Check sheet for the modelled part. Datum: model origin and axes. Units: mm. Face numbers are marked on the shaded views. Round coordinates to 2 decimals unless told otherwise and drop trailing zeros. Write each loop counter-clockwise with the first axis right and the second up, starting at its lowest first coordinate (ties: lowest second). Pieces come first, ordered by that corner, then holes. Notation, with made-up numbers: M 45.25,25.5 L 53.25,25.5 A18 ccw 53.25,49.5 Z; hole C 50.5,-20.75 d7. An arc over 180 degrees is marked long. Put each result on its own line as item: value.
Autodesk Inventor part; units mm, degrees
ref_plane "YZ Plane" through (0, 0, 0) normal (1, 0, 0) x (0, 1, 0)
ref_plane "XZ Plane" through (0, 0, 0) normal (0, 1, 0) x (-1, 0, 0)
ref_plane "XY Plane" through (0, 0, 0) normal (0, 0, 1) x (1, 0, 0)
sketch "Sketch1" plane through (0, 0, 0) normal (0, 1, 0) x (-1, 0, 0)
  line L0 (0, 55) -> (0, -55) construction
  line L1 (-12, 55) -> (-12, -55)
  line L2 (12, -55) -> (12, 55)
  arc A0 (12, 55) -> (-12, 55) centre (0, 55) ccw
  arc A1 (-12, -55) -> (12, -55) centre (0, -55) ccw
  line L3 (-19, 30) -> (-19, -30)
  line L4 (-19, -30) -> (19, -30)
  line L5 (19, -30) -> (19, 30)
  line L6 (19, 30) -> (-19, 30)
  line L7 (-19, 30) -> (19, -30) construction
  line L8 (-19, -30) -> (19, 30) construction
  point P0 (0, 0)
  point P1 (-12, 30)
  point P2 (-12, -30)
  point P3 (12, -30)
  point P4 (12, 30)
  dimension "d0" = 60
  dimension "d1" = 110
  dimension "d2" = 12
  dimension "d3" = 38
extrude "Extrusion1" add sketch "Sketch1" along normal blind 10
sketch "Sketch2" plane through (0, 10, 0) normal (0, 1, 0) x (1, 0, 0)
  line L0 (19, -30) -> (19, 30)
  line L1 (19, 30) -> (12, 30)
  line L2 (12, 30) -> (12, 55)
  arc A0 (12, 55) -> (-12, 55) centre (0, 55) ccw
  line L3 (-12, 55) -> (-12, 30)
  line L4 (-12, 30) -> (-19, 30)
  line L5 (-19, 30) -> (-19, -30)
  line L6 (-19, -30) -> (-12, -30)
  line L7 (-12, -30) -> (-12, -55)
  arc A1 (-12, -55) -> (12, -55) centre (0, -55) ccw
  line L8 (12, -55) -> (12, -30)
  line L9 (12, -30) -> (19, -30)
  line L10 (0, -28) -> (0, 28)
  line L11 (0, 0) -> (-19, 0)
  line L12 (-19, 30) -> (-19, -30)
  dimension "d6" = 56
hole "Hole1" at (0, 10, 28) at (0, 10, -28) direction (0, -1, 0) diameter 12 end through all
fillet "Fillet1" radius 3 8 edges at (19, 5, 30) (19, 5, -30) (12, 5, 30) (-19, 5, 30) (-12, 5, 30) (-19, 5, -30) (-12, 5, -30) (12, 5, -30)
sketch "Sketch3" plane through (0, 10, 0) normal (0, 1, 0) x (1, 0, 0)
  arc A0 (-12, -55) -> (12, -55) centre (0, -55) ccw
  arc A1 (12, 55) -> (-12, 55) centre (0, 55) ccw
  point P0 (0, 0)
hole "Hole2" at (0, 10, 55) at (0, 10, -55) direction (0, -1, 0) diameter 5.5 end through all
sketch "Sketch4" plane through (0, 10, 0) normal (0, 1, 0) x (1, 0, 0)
  circle A0 centre (0, 0) radius 3
  dimension "d22" = 6
extrude "Extrusion2" cut sketch "Sketch4" against normal blind 7.5
properties part number "04_Mieng_go_dem_lo_xo" material "Stainless Steel, Austenitic"
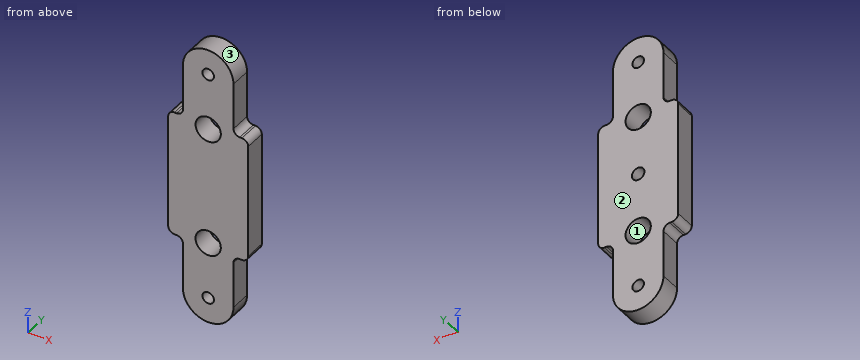
1. Cross-section at A-A (y = 4.5). Enter the section's corners in (x, z), then the cut area to 3 significant figures.
Computed values:
outline: M -19,-27 A3 ccw -16,-30 L -15,-30 A3 cw -12,-33 L -12,-55 A12 ccw 12,-55 L 12,-33 A3 cw 15,-30 L 16,-30 A3 ccw 19,-27 L 19,27 A3 ccw 16,30 L 15,30 A3 cw 12,33 L 12,55 A12 ccw -12,55 L -12,33 A3 cw -15,30 L -16,30 A3 ccw -19,27 Z; hole C 0,-28 d12; hole C 0,28 d12; hole C 0,0 d6; hole C 0,-55 d5.5; hole C 0,55 d5.5
area: 3,630 mm2
2. Scan lines: probe 1 along Z at (x, y) = (0, 7.25); probe 2 along X at (y, z) = (4.75, 0); probe 3 along X at (y, z) = (3, -55). Record each from-to range of solid material in increasing order.
Computed values:
probe 1: z = -67 to -57.75, -52.25 to -34, -22 to -3, 3 to 22, 34 to 52.25, 57.75 to 67
probe 2: x = -19 to -3, 3 to 19
probe 3: x = -12 to -2.75, 2.75 to 12
3. Cross-section at D-D (x = 8). Enter the section's corners in (y, z), then the cut area to 3 significant figures.
Computed values:
outline: M 0,-63.94 L 10,-63.94 L 10,63.94 L 0,63.94 Z
area: 1,280 mm2
4. Release check for a two-part mould opening along X. For the marked faces 1, 2 and 3 record: +X half, -X half, draft (parallel to the pull), parting line (faces both ways), or undercut.
Computed values:
face 1: undercut
face 2: draft
face 3: parting line
5. Depth check by flat-ended pin: pin 1 Ø9.5 at (x, z) = (0, 28) entering from -Y; pin 2 Ø1.1 at (x, y) = (-15.5, 3) entering from -Z; pin 3 Ø3 at (y, z) = (3, 46.5) entering from +X; pin 4 Ø4 at (y, z) = (5.5, -31.5) entering from +X. Enter the tip coordinate at first touch or a pass-through.
Computed values:
pin 1: passes through
pin 2: stops at z = -30
pin 3: stops at x = 12
pin 4: stops at x = 17.66
6. Cross-section at B-B (x = 0). Enter the section's corners in (y, z).
Computed values:
outline: M 0,-67 L 10,-67 L 10,-57.75 L 0,-57.75 Z; M 0,-52.25 L 10,-52.25 L 10,-34 L 0,-34 Z; M 0,-22 L 10,-22 L 10,-3 L 2.5,-3 L 2.5,3 L 10,3 L 10,22 L 0,22 Z; M 0,34 L 10,34 L 10,52.25 L 0,52.25 Z; M 0,57.75 L 10,57.75 L 10,67 L 0,67 Z
7. Cross-section at C-C (z = 0). Enter the section's corners in (x, y), then the cut area to 3 significant figures.
Computed values:
outline: M -19,0 L 19,0 L 19,10 L 3,10 L 3,2.5 L -3,2.5 L -3,10 L -19,10 Z
area: 335 mm2
